Could you check a few things on this model? Use its own coordinates, in mm. A direction names the side the tool comes from. Give positions to 0.01 mm unless a question says otherwise; leave off trailing zeros. Order: outer loops, then holes, each group sorted by start corner. A loop starts at its lowest first (then second) coordinate and runs counter-clockwise, first axis right, second up.
(1) Imagine slicing it at C-C, the plane z = 68. Write out the boundary of the cut face in (x, y).
(2) On a 3-axis mill with a long thin cutter (end or side, diameter ignored), from which of +Z, -Z, +X, -X, +Y, -Y can I reach the whole of each face in a straight line? I mean faces 5 (the flat face through (-15, -300, -3.175)), 6 (the flat face through (-13, -300, 0)), 7 (the flat face through (-185, -300, 126.873)), 8 (the flat face through (-457, -300, 0)), 9 (the flat face through (-440.563, -300, 59)). Say none if no direction works.
(3) Imagine slicing it at D-D, the plane y = -511. Write out the boundary of the cut face in (x, z) (3 decimals), then the cut area to 3 significant figures.
(4) If we mould it in two halves opening along X, with no side actions, what happens to faces 1 (the flat face through (-192, -300, 123.698)), 2 (the flat face through (-29.083, -300, 61)), 3 (the flat face through (-132, -609.092, 125)), 4 (the flat face through (-25.908, -300, 63))? For each: released by +X, released by -X, zero draft, split by the parting line, or undercut.
(5) Imagine slicing it at A-A, the plane y = -117. Write out the boundary of the cut face in (x, z) (3 decimals).
(6) Will these pins go through, and if not, where does the flat tip stop? pin 1 (3.5 mm diameter, centred on y = -192, z = 125.5, fed in from -X); pin 2 (4 mm diameter, centred on y = -523.5, z = 91.5, fed in from +X); pin 3 (8 mm diameter, centred on x = -456.946, y = -397.002, fed in from +Z).
(7) Imagine slicing it at B-B, the plane x = -271. Write out the boundary of the cut face in (y, z), then the cut area to 3 significant figures.
(8) If I drill on probe 1 along X at (y, z) = (-582.93, -2); probe 2 along X at (y, z) = (-371, 89.5); probe 3 along Z at (x, y) = (-429.5, -38.5), over which ranges is the centre line in solid material (lowest first)?
from build123d import *

# Parameters (mm, degrees)
F1_DEPTH = 609.092
F2_W     = 77
F2_H     = 339
F3_DEPTH = 25.4
F4_R     = 15.875
F5_DEPTH = 25.4
F7_D     = 7.14375


# Not quite as in the source:
# - a length typed as a fraction of an inch, garbled in the dataset ("3 / 203.2 mm" for 3/8 in), is restored


with BuildPart() as f1:
    # F0 (on Front) → F1 (new body)
    with BuildSketch(Plane.XZ):
        Polygon((0, -3.175), (0, 0), (-25.908, 0), (-25.908, 126.873), (-443.738, 126.873), (-443.738, 0), (-469.9, 0), (-469.9, -3.175), (-440.563, -3.175), (-440.563, 123.698), (-29.083, 123.698), (-29.083, -3.175), align=None)
    extrude(amount=F1_DEPTH)

    # F2 (on face) → F3 (cut)
    with BuildSketch(Plane.XY.offset(126.873)):
        with Locations((-334.88, -241.382)):
            Rectangle(F2_W, F2_H)
        with Locations((-244.88, -241.382)):
            Rectangle(F2_W, F2_H)
    extrude(amount=-F3_DEPTH, mode=Mode.SUBTRACT)

    # F4 (on face) → F5 (cut)
    with BuildSketch(Plane.XY.offset(126.873)):
        with Locations((-363.474, -544.068)):
            Circle(F4_R)
    extrude(amount=-F5_DEPTH, mode=Mode.SUBTRACT)

    # F7 (through all)
    with Locations(Plane.XY):
        with Locations((-456.946, -25.908), (-456.946, -212.09), (-456.946, -397.002), (-456.946, -582.93), (-13.208, -582.93), (-13.208, -397.002), (-13.208, -212.09), (-13.208, -25.908)):
            Hole(F7_D / 2)


solid = f1.part
Answer block:
1. outline: (-443.74, -609.09) - (-440.56, -609.09) - (-440.56, 0) - (-443.74, 0) - close; (-29.08, -609.09) - (-25.91, -609.09) - (-25.91, 0) - (-29.08, 0) - close
2. face 5: -Z, +X, -X, +Y, -Y
2. face 6: +Z, +X, +Y, -Y
2. face 7: +Z, +X, -X, +Y, -Y
2. face 8: +Z, -X, +Y, -Y
2. face 9: -Z, +Y, -Y
3. outline: (-469.9, -3.175) - (-440.563, -3.175) - (-440.563, 123.698) - (-29.083, 123.698) - (-29.083, -3.175) - (0, -3.175) - (0, 0) - (-25.908, 0) - (-25.908, 126.873) - (-443.738, 126.873) - (-443.738, 0) - (-469.9, 0) - close
3. area: 2,300 mm2
4. face 1: undercut
4. face 2: undercut
4. face 3: zero draft
4. face 4: released by +X
5. outline: (-469.9, -3.175) - (-440.563, -3.175) - (-440.563, 123.698) - (-373.38, 123.698) - (-373.38, 126.873) - (-443.738, 126.873) - (-443.738, 0) - (-469.9, 0) - close; (-296.38, 123.698) - (-283.38, 123.698) - (-283.38, 126.873) - (-296.38, 126.873) - close; (-206.38, 123.698) - (-29.083, 123.698) - (-29.083, -3.175) - (0, -3.175) - (0, 0) - (-25.908, 0) - (-25.908, 126.873) - (-206.38, 126.873) - close
6. pin 1: stops at x = -443.74
6. pin 2: stops at x = -25.91
6. pin 3: stops at z = 0
7. outline: (-609.09, 123.7) - (-410.88, 123.7) - (-410.88, 126.87) - (-609.09, 126.87) - close; (-71.88, 123.7) - (0, 123.7) - (0, 126.87) - (-71.88, 126.87) - close
7. area: 858 mm2
8. probe 1: x = -469.9 to -460.52, -453.37 to -440.56, -29.08 to -16.78, -9.64 to 0
8. probe 2: x = -443.74 to -440.56, -29.08 to -25.91
8. probe 3: z = 123.7 to 126.87
